Input: part model. Units: mm. Frame: model coordinates. A direction names the side the tool comes from. Coordinates: 2 decimals unless noted, no trailing zeros. Order: outer loops, then holes, each group sorted by start corner. A loop starts at its lowest first (then second) coordinate and runs counter-clockwise, first axis right, second up.
from build123d import *

# Parameters (mm, degrees)
SKETCH2_W                 = 70
SKETCH2_H                 = 40
LID_PLATE_DEPTH           = 3
SKETCH3_R                 = 2
PORT_BORE_DEPTH           = 3
SKETCH4_R                 = 2
CUT_EXTRUDE2_DEPTH        = 3
SKETCH5_R                 = 1.7
SCREW_CLEARANCE_DEPTH     = 3
SKETCH6_R                 = 1.7
CUT_EXTRUDE4_DEPTH        = 3
SKETCH7_R                 = 1.7
CUT_EXTRUDE5_DEPTH        = 3
SKETCH8_R                 = 1.7
CUT_EXTRUDE6_DEPTH        = 3
SNAP_BEAM_START           = -10
SKETCH9_W                 = 1.6
SKETCH9_H                 = 8
SNAP_BEAM_DEPTH           = 10
SNAP_HOOK_START           = -10
SKETCH10_W                = 0.5
SKETCH10_H                = 8
SNAP_HOOK_DEPTH           = 1.5
SKETCH11_W                = 2
SKETCH11_H                = 8
SNAP_RELEASE_ACCESS_DEPTH = 3
BOSS_EXTRUDE4_START       = -10
SKETCH12_W                = 1.6
SKETCH12_H                = 8
BOSS_EXTRUDE4_DEPTH       = 10
BOSS_EXTRUDE5_START       = -10
SKETCH13_W                = 0.5
SKETCH13_H                = 8
BOSS_EXTRUDE5_DEPTH       = 1.5
SKETCH14_W                = 2
SKETCH14_H                = 8
CUT_EXTRUDE8_DEPTH        = 3


with BuildPart() as part:
    # Sketch2 → Lid_plate (new body)
    with BuildSketch(Plane.XY):
        Rectangle(SKETCH2_W, SKETCH2_H)
    extrude(amount=LID_PLATE_DEPTH)

    # Sketch3 → Port_bore (cut)
    with BuildSketch(Plane.XY):
        with Locations((-15, 0)):
            Circle(SKETCH3_R)
    extrude(amount=PORT_BORE_DEPTH, mode=Mode.SUBTRACT)

    # Sketch4 → Cut-Extrude2 (cut)
    with BuildSketch(Plane.XY):
        with Locations((15, 0)):
            Circle(SKETCH4_R)
    extrude(amount=CUT_EXTRUDE2_DEPTH, mode=Mode.SUBTRACT)

    # Sketch5 → Screw_clearance (cut)
    with BuildSketch(Plane.XY):
        with Locations((-27, -12)):
            Circle(SKETCH5_R)
    extrude(amount=SCREW_CLEARANCE_DEPTH, mode=Mode.SUBTRACT)

    # Sketch6 → Cut-Extrude4 (cut)
    with BuildSketch(Plane.XY):
        with Locations((-27, 12)):
            Circle(SKETCH6_R)
    extrude(amount=CUT_EXTRUDE4_DEPTH, mode=Mode.SUBTRACT)

    # Sketch7 → Cut-Extrude5 (cut)
    with BuildSketch(Plane.XY):
        with Locations((27, -12)):
            Circle(SKETCH7_R)
    extrude(amount=CUT_EXTRUDE5_DEPTH, mode=Mode.SUBTRACT)

    # Sketch8 → Cut-Extrude6 (cut)
    with BuildSketch(Plane.XY):
        with Locations((27, 12)):
            Circle(SKETCH8_R)
    extrude(amount=CUT_EXTRUDE6_DEPTH, mode=Mode.SUBTRACT)

    # Sketch9 → Snap_beam (add)
    with BuildSketch(Plane.XY.offset(SNAP_BEAM_START)):
        with Locations((-29.8, 0)):
            Rectangle(SKETCH9_W, SKETCH9_H)
    extrude(amount=SNAP_BEAM_DEPTH)

    # Sketch10 → Snap_hook (add)
    with BuildSketch(Plane.XY.offset(SNAP_HOOK_START)):
        with Locations((-30.85, 0)):
            Rectangle(SKETCH10_W, SKETCH10_H)
    extrude(amount=SNAP_HOOK_DEPTH)

    # Sketch11 → Snap_release_access (cut)
    with BuildSketch(Plane.XY):
        with Locations((-27, 0)):
            Rectangle(SKETCH11_W, SKETCH11_H)
    extrude(amount=SNAP_RELEASE_ACCESS_DEPTH, mode=Mode.SUBTRACT)

    # Sketch12 → Boss-Extrude4 (add)
    with BuildSketch(Plane.XY.offset(BOSS_EXTRUDE4_START)):
        with Locations((29.8, 0)):
            Rectangle(SKETCH12_W, SKETCH12_H)
    extrude(amount=BOSS_EXTRUDE4_DEPTH)

    # Sketch13 → Boss-Extrude5 (add)
    with BuildSketch(Plane.XY.offset(BOSS_EXTRUDE5_START)):
        with Locations((30.85, 0)):
            Rectangle(SKETCH13_W, SKETCH13_H)
    extrude(amount=BOSS_EXTRUDE5_DEPTH)

    # Sketch14 → Cut-Extrude8 (cut)
    with BuildSketch(Plane.XY):
        with Locations((27, 0)):
            Rectangle(SKETCH14_W, SKETCH14_H)
    extrude(amount=CUT_EXTRUDE8_DEPTH, mode=Mode.SUBTRACT)


solid = part.part
Item 1: Pin query (flat end, axial travel): pin 1 Ø8 at (x, y) = (-5.5, -13.5) entering from -Z; pin 2 Ø2.5 at (y, z) = (-2, -6) entering from +X; pin 3 Ø6.5 at (y, z) = (-1.5, -5.5) entering from +X; pin 4 Ø2 at (x, y) = (-27, -12) entering from +Z. Return the tip coordinate at first contact, or that it passes through.
Response values:
pin 1: stops at z = 0
pin 2: stops at x = 30.6
pin 3: stops at x = 31.1
pin 4: passes through
Item 2: Cut plane B-B on z = 2. Count the separate pieces of the cut face and the enclosed holes in it, then the cut area to 3 significant figures.
Response values:
separate pieces: 1
enclosed holes: 8
area: 2,710 mm2
Item 3: Cut plane A-A on x = 27. Return loops of the section in (y, z).
Response values:
outline: (-20, 0) - (-13.7, 0) - (-13.7, 3) - (-20, 3) - close; (-10.3, 0) - (-4, 0) - (-4, 3) - (-10.3, 3) - close; (4, 0) - (10.3, 0) - (10.3, 3) - (4, 3) - close; (13.7, 0) - (20, 0) - (20, 3) - (13.7, 3) - close
Item 4: Cut plane C-C on y = 12. Return loops of the section in (x, z).
Response values:
outline: (-35, 0) - (-28.7, 0) - (-28.7, 3) - (-35, 3) - close; (-25.3, 0) - (25.3, 0) - (25.3, 3) - (-25.3, 3) - close; (28.7, 0) - (35, 0) - (35, 3) - (28.7, 3) - close
Item 5: Access query for faces 1 (the face through (28, 0, 1)), 2 (the face through (-30, 4, -5)), 3 (the face through (0, 0, 3)), 4 (the face through (0, -20, 1)), 5 (the face through (29, 0, -5)). Directions: +Z, -Z, +X, -X, +Y, -Y. A direction counts if a zero-diameter tool reaches every point of the face in a straight line with its end or side. Return the directions, or none.
Response values:
face 1: +Z, -Z
face 2: -Z, +X, -X, +Y
face 3: +Z, +X, -X, +Y, -Y
face 4: +Z, -Z, +X, -X, -Y
face 5: -Z, +Y, -Y
Item 6: Ray query, probe 1 along Y at (x, z) = (27, 0.95); probe 2 along X at (y, z) = (-2, -5.5); probe 3 along Z at (x, y) = (7.5, -3.5). Return the intervals inside material, ascending.
Response values:
probe 1: y = -20 to -13.7, -10.3 to -4, 4 to 10.3, 13.7 to 20
probe 2: x = -30.6 to -29, 29 to 30.6
probe 3: z = 0 to 3
Item 7: Cut plane D-D on x = -15. Return loops of the section in (y, z), then the cut area to 3 significant figures.
Response values:
outline: (-20, 0) - (-2, 0) - (-2, 3) - (-20, 3) - close; (2, 0) - (20, 0) - (20, 3) - (2, 3) - close
area: 108 mm2
Item 8: Draft query along X for faces 6 (the face through (30.6, 0, -4)), 7 (the face through (-31.1, 0, -9)), 8 (the face through (-25.43, 11.35, 1.48)), 9 (the face through (30, 0, -10)). Return one class per face: pulls with the +X half, pulls with the -X half, needs draft (parallel to the pull), parting line crosses it, or undercut.
Response values:
face 6: pulls with the +X half
face 7: pulls with the -X half
face 8: undercut
face 9: needs draft
